```python
from build123d import *

# Parameters (mm, degrees)
SKETCH1_W           = 150
SKETCH1_H           = 80
BOSS_EXTRUDE1_DEPTH = 15
CUT_EXTRUDE1_REACH  = 88.313
SKETCH2_R           = 3
SKETCH2_R_2         = 5.5
SKETCH3_R           = 11.1
SKETCH3_R_2         = 10
CUT_EXTRUDE2_DEPTH  = 8
SKETCH5_R           = 5
CUT_EXTRUDE4_DEPTH  = 4
SKETCH6_R           = 2.5
CUT_EXTRUDE5_DEPTH  = 10
SKETCH7_R           = 2.5
CUT_EXTRUDE6_DEPTH  = 10
SKETCH8_R           = 2.5
CUT_EXTRUDE7_DEPTH  = 10


with BuildPart() as part:
    # Sketch1 → Boss-Extrude1 (new body)
    with BuildSketch(Plane.XY):
        Rectangle(SKETCH1_W, SKETCH1_H)
    extrude(amount=BOSS_EXTRUDE1_DEPTH)

    # Sketch2 → Cut-Extrude1 (cut, up to next)
    with BuildSketch(Plane.XY.offset(15), mode=Mode.PRIVATE) as cut_extrude1_sk1:
        with Locations((-50, 0)):
            Circle(SKETCH2_R)
    cut_extrude1_tool1 = extrude(cut_extrude1_sk1.sketch, amount=-CUT_EXTRUDE1_REACH, mode=Mode.PRIVATE) & part.part
    # Sketch2 → Cut-Extrude1 (cut, up to next)
    with BuildSketch(Plane.XY.offset(15), mode=Mode.PRIVATE) as cut_extrude1_sk2:
        with Locations((50, 0)):
            Circle(SKETCH2_R)
    cut_extrude1_tool2 = extrude(cut_extrude1_sk2.sketch, amount=-CUT_EXTRUDE1_REACH, mode=Mode.PRIVATE) & part.part
    # Sketch2 → Cut-Extrude1 (cut, up to next)
    with BuildSketch(Plane.XY.offset(15), mode=Mode.PRIVATE) as cut_extrude1_sk3:
        Circle(SKETCH2_R_2)
    cut_extrude1_tool3 = extrude(cut_extrude1_sk3.sketch, amount=-CUT_EXTRUDE1_REACH, mode=Mode.PRIVATE) & part.part
    add(cut_extrude1_tool1.solids().sort_by_distance((-50, 0, 15))[0], mode=Mode.SUBTRACT)
    add(cut_extrude1_tool2.solids().sort_by_distance((50, 0, 15))[0], mode=Mode.SUBTRACT)
    add(cut_extrude1_tool3.solids().sort_by_distance((0, 0, 15))[0], mode=Mode.SUBTRACT)

    # Sketch3 → Cut-Extrude2 (cut)
    with BuildSketch(Plane.XY.offset(15)):
        Circle(SKETCH3_R)
        with Locations((-50, 0)):
            Circle(SKETCH3_R_2)
        with Locations((50, 0)):
            Circle(SKETCH3_R_2)
    extrude(amount=-CUT_EXTRUDE2_DEPTH, mode=Mode.SUBTRACT)

    # Sketch5 → Cut-Extrude4 (cut)
    with BuildSketch(Plane(origin=(0, 0, 0), x_dir=(-1, 0, 0), z_dir=(0, 0, -1))):
        with Locations((-50, 0)):
            Circle(SKETCH5_R)
        with Locations((50, 0)):
            Circle(SKETCH5_R)
    extrude(amount=-CUT_EXTRUDE4_DEPTH, mode=Mode.SUBTRACT)

    # Sketch6 → Cut-Extrude5 (cut)
    with BuildSketch(Plane.ZY.offset(75)):
        with Locations((8, 1)):
            Circle(SKETCH6_R)
    cut_extrude5 = extrude(amount=-CUT_EXTRUDE5_DEPTH, mode=Mode.SUBTRACT)

    # Mirror1: Cut-Extrude5 across plane
    add(cut_extrude5.mirror(Plane(origin=(0, 0, 0), x_dir=(0, 0, 1), z_dir=(1, 0, 0))), mode=Mode.SUBTRACT)

    # Sketch7 → Cut-Extrude6 (cut)
    with BuildSketch(Plane.XZ.offset(40)):
        with Locations((-62, 8)):
            Circle(SKETCH7_R)
        with Locations(Location((62, 8, 0), (0, 0, 180))):
            Circle(SKETCH7_R)
    extrude(amount=-CUT_EXTRUDE6_DEPTH, mode=Mode.SUBTRACT)

    # Sketch8 → Cut-Extrude7 (cut)
    with BuildSketch(Plane(origin=(0, 40, 0), x_dir=(1, 0, 0), z_dir=(0, 1, 0))):
        with Locations(Location((0, -8, 0), (0, 0, 180))):
            Circle(SKETCH8_R)
    extrude(amount=-CUT_EXTRUDE7_DEPTH, mode=Mode.SUBTRACT)


solid = part.part
```
Geometry check sheet. Reference: the model listing, model coordinates, mm. A direction names the side the tool comes from. Coordinates: 2 decimals unless noted, no trailing zeros. Loops run counter-clockwise (first coordinate to the right, second up) from the corner with the lowest first, then second, coordinate; pieces in that order, holes last.
Item 1: Sectioned sample at A-A, the plane x = 0. Record the boundary of the cut face in (y, z).
Item 2: Go/stop test with flat-tipped pins: pin 1 Ø18 at (x, y) = (-50, 0) entering from +Z; pin 2 Ø8 at (x, y) = (10, -19.5) entering from -Z; pin 3 Ø5 at (x, y) = (49, 0.5) entering from -Z; pin 4 Ø3 at (y, z) = (1, 8) entering from -X. Record where each tip stops, or that it passes through.
Item 3: Thickness scan on line 1 (Y direction, x = 46, z = 3.25); line 2 (X direction, y = 31, z = 8.25); line 3 (X direction, y = 2, z = 6.75). Record the ranges inside material, lowest first.
Item 4: Sectioned sample at B-B, the plane x = -62. Record the boundary of the cut face in (y, z).
Item 5: Access from +Z, -Z, +X, -X, +Y, -Y to the whole of each face (thin tool, end or side, straight path). Record for faces 1 (the face through (65, 1, 8)), 2 (the face through (0.54, 35.07, 5.56)), 3 (the face through (-70.07, 1.751, 10.385)), 4 (the face through (62, -30, 8)), 5 (the face through (-3, 5, 7)).
Item 6: Release check for a two-part mould opening along X. For faces 6 (the face through (75, -1, 6)), 7 (the face through (-53, 0, 6)), 8 (the face through (-1, 40, 4)) record: released by +X, released by -X, zero draft, split by the parting line, or undercut.
Item 7: Sectioned sample at C-C, the plane x = 51. Record the boundary of the cut face in (y, z), then the cut area to 3 significant figures.
Check result:
1. outline: (-40, 0) - (-5.5, 0) - (-5.5, 7) - (-11.1, 7) - (-11.1, 15) - (-40, 15) - close; (5.5, 0) - (40, 0) - (40, 5.5) - (30, 5.5) - (30, 10.5) - (40, 10.5) - (40, 15) - (11.1, 15) - (11.1, 7) - (5.5, 7) - close
2. pin 1: stops at z = 7
2. pin 2: stops at z = 0
2. pin 3: stops at z = 4
2. pin 4: stops at x = -65
3. line 1: y = -40 to -3, 3 to 40
3. line 2: x = -75 to -2.49, 2.49 to 75
3. line 3: x = -65 to -52.24, -47.76 to -5.12, 5.12 to 47.76, 52.24 to 65
4. outline: (-40, 0) - (40, 0) - (40, 15) - (-40, 15) - (-40, 10.5) - (-30, 10.5) - (-30, 5.5) - (-40, 5.5) - close
5. face 1: +X
5. face 2: +Y
5. face 3: -X
5. face 4: -Y
5. face 5: +Z
6. face 6: released by +X
6. face 7: undercut
6. face 8: zero draft
7. outline: (-40, 0) - (-4.9, 0) - (-4.9, 4) - (-2.83, 4) - (-2.83, 7) - (-9.95, 7) - (-9.95, 15) - (-40, 15) - close; (2.83, 4) - (4.9, 4) - (4.9, 0) - (40, 0) - (40, 15) - (9.95, 15) - (9.95, 7) - (2.83, 7) - close
7. area: 985 mm2
